```python
from build123d import *

# Parameters (mm, degrees)
CHAMFER_1_SIZE = 0.5


with BuildPart() as part:
    # 草图1 → 旋转1 (revolve)
    with BuildSketch(Plane.XY, mode=Mode.PRIVATE) as revolve_1_sk:
        with BuildLine():
            Line((-3, 7.05), (3, 7.05))
            Line((3, 7.05), (3, 15))
            Line((3, 15), (2.5, 15))
            Line((2.5, 15), (1.299038106, 12.919872981))
            ThreePointArc((1.299038106, 12.919872981), (0, 12.169872981), (-1.299038106, 12.919872981))
            Line((-1.299038106, 12.919872981), (-2.5, 15))
            Line((-2.5, 15), (-3, 15))
            Line((-3, 15), (-3, 7.05))
        make_face()
    revolve(revolve_1_sk.sketch.rotate(Axis((-10.233108396, 0, 0), (1, 0, 0)), 90), axis=Axis((-10.233108396, 0, 0), (1, 0, 0)))

    # 倒角1
    chamfer_1_edges = [part.edges().sort_by_distance(p)[0] for p in [
        (3, 0, -7.05),
        (-3, 0, -7.05),
    ]]
    chamfer(chamfer_1_edges, length=CHAMFER_1_SIZE)


solid = part.part
```
Source: CAD feature listing. Evaluate the final solid. Frame: model axes, mm. A direction names the side the tool comes from. Give positions to 0.01 mm unless a question says otherwise; leave off trailing zeros. Write each loop counter-clockwise with the first axis right and the second up, starting at its lowest first coordinate (ties: lowest second). Pieces come first, ordered by that corner, then holes.
1. First-contact query: pin 1 (3 mm diameter, centred on x = 2, z = -12, fed in from +Y). Flat tip, straight axial feed; report the tip coordinate or a pass-through.
2. Access query for faces 1 (the face through (-3, -7, -4)), 2 (the face through (-1.374, -12.939, -1.699)). Directions: +Z, -Z, +X, -X, +Y, -Y. A direction counts if a zero-diameter tool reaches every point of the face in a straight line with its end or side. Return the directions, or none.
3. Section query A-A (z = 0). Return the cut outline in (x, y).
4. Section query C-C (x = 0.4). Return the cut outline in (y, z).
5. Pull-direction query (Z, two-part tool) for faces 3 (the face through (0.04, 6.88, -1.53)), 4 (the face through (3, -7, 4)), 5 (the face through (2.75, -12.65, 8.06)); classes: +Z half, -Z half, draft (parallel to the pull), parting line (faces both ways), or undercut.
6. Material intervals for line 1 along Y through (x, z) = (1.25, 0); line 2 along Y through (x, z) = (-1.65, -2); line 3 along Z through (x, y) = (-1.8, -0.75), sorted ascending.
Output values:
1. pin 1: stops at y = 10.63
2. face 1: +Z, -Z, -X, +Y, -Y
2. face 2: none
3. outline: (-3, -15) - (-2.5, -15) - (-1.3, -12.92) arc R1.5 cw to (1.3, -12.92) - (2.5, -15) - (3, -15) - (3, -7.55) - (2.5, -7.05) - (-2.5, -7.05) - (-3, -7.55) - close; (-3, 7.55) - (-2.5, 7.05) - (2.5, 7.05) - (3, 7.55) - (3, 15) - (2.5, 15) - (1.3, 12.92) arc R1.5 cw to (-1.3, 12.92) - (-2.5, 15) - (-3, 15) - close
4. outline: circle Ø24.45 at (0, 0); hole circle Ø14.1 at (0, 0)
5. face 3: undercut
5. face 4: draft
5. face 5: parting line
6. line 1: y = -12.84 to -7.05, 7.05 to 12.84
6. line 2: y = -13.38 to -6.76, 6.76 to 13.38
6. line 3: z = -13.77 to -7.01, 7.01 to 13.77
